Verification items for the finished model (mm, model axes). Face numbers are marked on the shaded views. A direction names the side the tool comes from. Give positions to 0.01 mm unless a question says otherwise; leave off trailing zeros. Order: outer loops, then holes, each group sorted by start corner. A loop starts at its lowest first (then second) coordinate and runs counter-clockwise, first axis right, second up. Notation, with made-up numbers: (35.5, 10.5) -> (49.5, 10.5) arc R37 cw to (49.5, 47.5) -> close; hole circle Ø5 at (4, 76.25). An arc over 180 degrees is marked (long way). One line per question, with ' | ' between items. Start each with the question number.
Q1. Section check B-B on z = 31. Record the cut outline in (x, y).
Q2. Access from +Z, -Z, +X, -X, +Y, -Y to the whole of each face (thin tool, end or side, straight path). Record for the marked faces 4, 5, 6 and 7.
Q3. Material ranges on probe 1 along Z at (x, y) = (13, -51); probe 2 along Y at (x, z) = (23.5, 45.5); probe 3 along Y at (x, z) = (11, 44.5), recorded low to high. Write a range as [from, to].
Q4. Section check C-C on y = 17. Record the cut outline in (x, z), plus the area to 3 significant figures.
Q5. Section check A-A on y = -8.5. Record the cut outline in (x, z).
Q6. Mould release check, pull along Z, two halves, no side actions. Record for the marked faces 1, 2 and 3: released by +Z, released by -Z, zero draft, split by the parting line, or undercut.
Q7. Section check D-D on y = 2. Record the cut outline in (x, z), plus the area to 3 significant figures.
Q8. Go/stop test with flat-tipped pins: pin 1 (8 mm diameter, centred on x = 11, z = 49.5, fed in from +Y); pin 2 (6 mm diameter, centred on y = -12.5, z = 31.5, fed in from -X); pin 3 (3.5 mm diameter, centred on x = 21, y = -57.5, fed in from +Z); pin 4 (5 mm diameter, centred on x = 19, y = -12.5, fed in from -Z). Record where each tip stops, or that it passes through.
from build123d import *

# Parameters (mm, degrees)
SKETCH1_R                                        = 0.9
SKETCH1_W                                        = 12
SKETCH1_H                                        = 23
BOSS_EXTRUDE1_DEPTH                              = 15
CBORE_FOR_M4_PAN_HEAD_MACHINE_SCREW2_D           = 4.5
CBORE_FOR_M4_PAN_HEAD_MACHINE_SCREW2_CBORE_D     = 9
CBORE_FOR_M4_PAN_HEAD_MACHINE_SCREW2_CBORE_DEPTH = 3.1
CUT_EXTRUDE2_DEPTH                               = 4
SKETCH11_W                                       = 38.11
SKETCH11_H                                       = 57
CUT_EXTRUDE3_DEPTH                               = 9
FILLET3_R                                        = 6
FILLET4_R                                        = 4
BOSS_EXTRUDE2_DEPTH                              = 10
FILLET2_R                                        = 4
SKETCH14_W                                       = 40.700591816
SKETCH14_H                                       = 70
CUT_EXTRUDE4_DEPTH                               = 4


with BuildPart() as part:
    # Sketch1 → Boss-Extrude1 (new body)
    with BuildSketch(Plane(origin=(0, 0, 0), x_dir=(0, 0, -1), z_dir=(1, 0, 0))):
        with BuildLine():
            Line((-58.460295908, -42.411439664), (-41.718412731, -42.411439664))
            ThreePointArc((-41.718412731, -42.411439664), (-25.860295908, -43.911439664), (-41.718412731, -45.411439664))
            Line((-41.718412731, -45.411439664), (-58.460295908, -45.411439664))
            Line((-58.460295908, -45.411439664), (-58.460295908, -58.911439664))
            Line((-58.460295908, -58.911439664), (-20.350295908, -58.911439664))
            Line((-20.350295908, -58.911439664), (-20.350295908, -16.911439664))
            Line((-20.350295908, -16.911439664), (13.649704092, -16.911439664))
            Line((13.649704092, -16.911439664), (13.649704092, 37.088560336))
            Line((13.649704092, 37.088560336), (-10.350295908, 37.088560336))
            Line((-10.350295908, 37.088560336), (-10.350295908, -1.911439664))
            Line((-10.350295908, -1.911439664), (-58.460295908, -1.911439664))
            Line((-58.460295908, -1.911439664), (-58.460295908, -28.911439664))
            Line((-58.460295908, -28.911439664), (-58.460295908, -42.411439664))
        make_face()
        with Locations((1.649704092, 34.088560336)):
            Circle(SKETCH1_R, mode=Mode.SUBTRACT)
        with Locations((1.649704092, 5.088560336)):
            Circle(SKETCH1_R, mode=Mode.SUBTRACT)
        with Locations((1.649704092, 19.588560336)):
            Rectangle(SKETCH1_W, SKETCH1_H, mode=Mode.SUBTRACT)
    extrude(amount=BOSS_EXTRUDE1_DEPTH)

    # CBORE for M4 Pan Head Machine Screw2 (through all)
    with Locations(Plane(origin=(0, -58.911439664, 0), x_dir=(-1, 0, 0), z_dir=(0, -1, 0))):
        with Locations((-12, -52.560295908)):
            CounterBoreHole(CBORE_FOR_M4_PAN_HEAD_MACHINE_SCREW2_D / 2, CBORE_FOR_M4_PAN_HEAD_MACHINE_SCREW2_CBORE_D / 2, CBORE_FOR_M4_PAN_HEAD_MACHINE_SCREW2_CBORE_DEPTH)

    # Sketch7 → Cut-Extrude2 (cut)
    with BuildSketch(Plane(origin=(0, -1.911439664, 0), x_dir=(1, 0, 0), z_dir=(0, 1, 0))):
        Polygon((15.553380664, -50.516569118), (12.006771014, -48.461114589), (8.45339035, -50.504841379), (8.446619336, -54.604022698), (11.993228986, -56.659477227), (15.54660965, -54.615750437), align=None)
    extrude(amount=-CUT_EXTRUDE2_DEPTH, mode=Mode.SUBTRACT)

    # Sketch11 → Cut-Extrude3 (cut)
    with BuildSketch(Plane.ZY):
        with Locations((39.405295908, -30.411439664)):
            Rectangle(SKETCH11_W, SKETCH11_H)
    extrude(amount=-CUT_EXTRUDE3_DEPTH, mode=Mode.SUBTRACT)

    # Fillet3
    fillet3_edges = [part.edges().sort_by_distance(p)[0] for p in [
        (7.5, 37.088560336, 10.350295908),
        (7.5, 37.088560336, -13.649704092),
    ]]
    fillet(fillet3_edges, radius=FILLET3_R)

    # Fillet4
    # the kernel refuses this fillet: 4 mm, written as the material it takes off along each edge
    with BuildSketch(Plane(origin=(0, 31.088560336, 10.350295908), x_dir=(0, 0, -1), z_dir=(0, -1, 0))) as fillet4_piece_1:
        with BuildLine():
            CenterArc((FILLET4_R, FILLET4_R), FILLET4_R, 180, 90)
            Line((0, FILLET4_R), (0, 0))
            Line((0, 0), (FILLET4_R, 0))
        make_face()
    extrude(amount=33, mode=Mode.SUBTRACT)
    with BuildSketch(Plane(origin=(15, 31.088560336, 10.350295908), x_dir=(0, 0, -1), z_dir=(0, -1, 0))) as fillet4_piece_2:
        with BuildLine():
            CenterArc((FILLET4_R, -FILLET4_R), FILLET4_R, 90, 90)
            Line((0, -FILLET4_R), (0, 0))
            Line((0, 0), (FILLET4_R, 0))
        make_face()
    extrude(amount=33, mode=Mode.SUBTRACT)
    with BuildSketch(Plane(origin=(0, 37.088560336, -7.649704092), x_dir=(1, 0, 0), z_dir=(0, 0, 1))) as fillet4_piece_3:
        with BuildLine():
            CenterArc((FILLET4_R, -FILLET4_R), FILLET4_R, 90, 90)
            Line((0, -FILLET4_R), (0, 0))
            Line((0, 0), (FILLET4_R, 0))
        make_face()
    extrude(amount=12, mode=Mode.SUBTRACT)
    with BuildSketch(Plane(origin=(0, 31.088560336, -7.649704092), x_dir=(0, 1, 0), z_dir=(0, 0, 1))) as fillet4_piece_4:
        with BuildLine():
            CenterArc((6 - FILLET4_R, -FILLET4_R), FILLET4_R, 0, 90)
            Line((6, -FILLET4_R), (6, 0))
            Line((6, 0), (6 - FILLET4_R, 0))
        make_face()
    revolve(axis=Axis((0, 31.088560336, -7.649704092), (-1, 0, 0)), revolution_arc=90, mode=Mode.SUBTRACT)
    with BuildSketch(Plane(origin=(0, 31.088560336, 4.350295908), x_dir=(0, 1, 0), z_dir=(0, 0, -1))) as fillet4_piece_5:
        with BuildLine():
            CenterArc((6 - FILLET4_R, FILLET4_R), FILLET4_R, 270, 90)
            Line((6, FILLET4_R), (6, 0))
            Line((6, 0), (6 - FILLET4_R, 0))
        make_face()
    revolve(axis=Axis((0, 31.088560336, 4.350295908), (1, 0, 0)), revolution_arc=90, mode=Mode.SUBTRACT)
    with BuildSketch(Plane(origin=(15, 37.088560336, -7.649704092), x_dir=(-1, 0, 0), z_dir=(0, 0, 1))) as fillet4_piece_6:
        with BuildLine():
            CenterArc((FILLET4_R, FILLET4_R), FILLET4_R, 180, 90)
            Line((0, FILLET4_R), (0, 0))
            Line((0, 0), (FILLET4_R, 0))
        make_face()
    extrude(amount=12, mode=Mode.SUBTRACT)
    with BuildSketch(Plane(origin=(15, 31.088560336, -7.649704092), x_dir=(0, 1, 0), z_dir=(0, 0, 1))) as fillet4_piece_7:
        with BuildLine():
            CenterArc((6 - FILLET4_R, FILLET4_R), FILLET4_R, 270, 90)
            Line((6 - FILLET4_R, 0), (6, 0))
            Line((6, 0), (6, FILLET4_R))
        make_face()
    revolve(axis=Axis((15, 31.088560336, -7.649704092), (-1, 0, 0)), revolution_arc=90, mode=Mode.SUBTRACT)
    with BuildSketch(Plane(origin=(15, 31.088560336, 4.350295908), x_dir=(0, 1, 0), z_dir=(0, 0, -1))) as fillet4_piece_8:
        with BuildLine():
            CenterArc((6 - FILLET4_R, -FILLET4_R), FILLET4_R, 0, 90)
            Line((6 - FILLET4_R, 0), (6, 0))
            Line((6, 0), (6, -FILLET4_R))
        make_face()
    revolve(axis=Axis((15, 31.088560336, 4.350295908), (1, 0, 0)), revolution_arc=90, mode=Mode.SUBTRACT)
    with BuildSketch(Plane(origin=(0, -26.911439664, -13.649704092), x_dir=(0, 0, 1), z_dir=(0, 1, 0))) as fillet4_piece_9:
        with BuildLine():
            CenterArc((FILLET4_R, FILLET4_R), FILLET4_R, 180, 90)
            Line((0, FILLET4_R), (0, 0))
            Line((0, 0), (FILLET4_R, 0))
        make_face()
    extrude(amount=58, mode=Mode.SUBTRACT)
    with BuildSketch(Plane(origin=(-10, -16.911439664, -13.649704092), x_dir=(0, 1, 0), z_dir=(1, 0, 0))) as fillet4_piece_10:
        with BuildLine():
            CenterArc((FILLET4_R, FILLET4_R), FILLET4_R, 180, 90)
            Line((0, FILLET4_R), (0, 0))
            Line((0, 0), (FILLET4_R, 0))
        make_face()
    extrude(amount=35, mode=Mode.SUBTRACT)
    with BuildSketch(Plane(origin=(15, -26.911439664, -13.649704092), x_dir=(0, 0, 1), z_dir=(0, 1, 0))) as fillet4_piece_11:
        with BuildLine():
            CenterArc((FILLET4_R, -FILLET4_R), FILLET4_R, 90, 90)
            Line((0, -FILLET4_R), (0, 0))
            Line((0, 0), (FILLET4_R, 0))
        make_face()
    extrude(amount=58, mode=Mode.SUBTRACT)

    # Sketch13 → Boss-Extrude2 (add)
    with BuildSketch(Plane(origin=(15, 0, 0), x_dir=(0, 0, -1), z_dir=(1, 0, 0))):
        with BuildLine():
            Line((-41.718412731, -42.411439664), (-50.089354319, -42.411439664))
            Line((-50.089354319, -42.411439664), (-50.089354319, -29.340681858))
            Line((-50.089354319, -29.340681858), (-20.350295908, -29.340681858))
            Line((-20.350295908, -29.340681858), (-20.350295908, -58.911439664))
            Line((-20.350295908, -58.911439664), (-49.206193942, -58.911439664))
            Line((-49.206193942, -58.911439664), (-49.206193942, -55.811439664))
            Line((-49.206193942, -55.811439664), (-52.560295908, -55.811439664))
            Line((-52.560295908, -55.811439664), (-50.089354319, -45.411439664))
            Line((-50.089354319, -45.411439664), (-41.718412731, -45.411439664))
            ThreePointArc((-41.718412731, -45.411439664), (-25.860295908, -43.911439664), (-41.718412731, -42.411439664))
        make_face()
    extrude(amount=BOSS_EXTRUDE2_DEPTH)

    # Fillet2
    # the kernel refuses this fillet: 4 mm, written as the material it adds along each edge
    with BuildSketch(Plane(origin=(9, -1.911439664, 20.350295908), x_dir=(-1, 0, 0), z_dir=(0, -1, 0))) as fillet2_piece_1:
        with BuildLine():
            CenterArc((FILLET2_R, -FILLET2_R), FILLET2_R, 90, 90)
            Line((0, -FILLET2_R), (0, 0))
            Line((0, 0), (FILLET2_R, 0))
        make_face()
    extrude(amount=15)
    # the kernel refuses this fillet: 4 mm, written as the material it takes off along each edge
    with BuildSketch(Plane(origin=(35, -58.911439664, 20.350295908), x_dir=(0, 1, 0), z_dir=(-1, 0, 0))) as fillet2_2_piece_1:
        with BuildLine():
            CenterArc((FILLET2_R, -FILLET2_R), FILLET2_R, 90, 90)
            Line((0, -FILLET2_R), (0, 0))
            Line((0, 0), (FILLET2_R, 0))
        make_face()
    extrude(amount=36, mode=Mode.SUBTRACT)
    with BuildSketch(Plane(origin=(0, 8.088560336, 20.350295908), x_dir=(0, 0, -1), z_dir=(0, -1, 0))) as fillet2_2_piece_2:
        with BuildLine():
            CenterArc((FILLET2_R, FILLET2_R), FILLET2_R, 180, 90)
            Line((0, FILLET2_R), (0, 0))
            Line((0, 0), (FILLET2_R, 0))
        make_face()
    extrude(amount=35, mode=Mode.SUBTRACT)
    with BuildSketch(Plane(origin=(15, -55.811439664, 52.560295908), x_dir=(0, 0, -1), z_dir=(1, 0, 0))) as fillet2_2_piece_3:
        with BuildLine():
            CenterArc((4.979691241, 3.654785836), FILLET2_R, 166.634871225, 79.386408779)
            Line((1.088024265, 4.579409084), (0, 0))
            Line((0, 0), (3.354101966, 0))
        make_face()
    extrude(amount=21.76721727, mode=Mode.SUBTRACT)
    with BuildSketch(Plane(origin=(15, -29.340681858, 20.350295908), x_dir=(0, -1, 0), z_dir=(1, 0, 0)), Plane(origin=(15, -29.340681858, 50.089354319), x_dir=(0, 0, -1), z_dir=(1, 0, 0))) as fillet2_2_piece_4:
        with BuildLine():
            CenterArc((FILLET2_R, -FILLET2_R), FILLET2_R, 90, 90)
            Line((0, -FILLET2_R), (0, 0))
            Line((0, 0), (FILLET2_R, 0))
        make_face()
    extrude(amount=20, mode=Mode.SUBTRACT)

    # Sketch14 → Cut-Extrude4 (cut)
    with BuildSketch(Plane(origin=(15, 0, 0), x_dir=(0, 0, -1), z_dir=(1, 0, 0))):
        with Locations((0, 5.659318142)):
            Rectangle(SKETCH14_W, SKETCH14_H)
    extrude(amount=-CUT_EXTRUDE4_DEPTH, mode=Mode.SUBTRACT)


solid = part.part
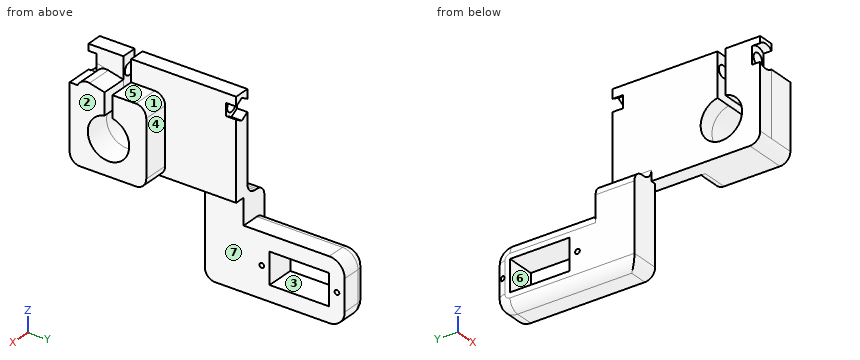
Filled in:
1) outline: (9, -58.91) -> (25, -58.91) -> (25, -51.38) -> (9, -51.38) -> close; (9, -36.44) -> (25, -36.44) -> (25, -29.34) -> (15, -29.34) -> (15, -1.91) -> (9, -1.91) -> close
2) face 4: +Z, -Z, +X, +Y | face 5: +Z, +X, +Y | face 6: +X, -X | face 7: -Z, +X, +Y, -Y
3) probe 1: [20.35, 30.15], [37.57, 50.54], [54.58, 58.46] | probe 2: [-58.91, -45.41], [-42.41, -29.34] | probe 3: [-58.91, -45.41], [-42.41, -1.91]
4) outline: (0, -9.65) arc R4 ccw to (4, -13.65) -> (11, -13.65) -> (11, -7.65) -> (0, -7.65) -> close; (0, 4.35) -> (11, 4.35) -> (11, 10.35) -> (4, 10.35) arc R4 ccw to (0, 6.35) -> close | area: 125 mm²
5) outline: (0, -9.65) arc R4 ccw to (4, -13.65) -> (11, -13.65) -> (11, 20.35) -> (15, 20.35) -> (15, 58.46) -> (9, 58.46) -> (9, 24.35) arc R4 cw to (5, 20.35) -> (4, 20.35) arc R4 ccw to (0, 16.35) -> close; hole circle Ø4.5 at (12, 52.56)
6) face 1: released by +Z | face 2: zero draft | face 3: undercut
7) outline: (0, -9.65) arc R4 ccw to (4, -13.65) -> (11, -13.65) -> (11, 10.35) -> (4, 10.35) arc R4 ccw to (0, 6.35) -> close | area: 257 mm²
8) pin 1: y = -1.91 | pin 2: x = 9 | pin 3: z = 49.34 | pin 4: through
